Design review of the part shown in the three views and the two pictorial views. Dimensions are in mm from the part's minimum x, y and z. Coordinates: 2 decimals unless noted, no trailing zeros. Write each loop counter-clockwise with the first axis right and the second up, starting at its lowest first coordinate (ties: lowest second). Pieces come first, ordered by that corner, then holes. Notation, with made-up numbers: (-24.5, 27) -> (30.5, 27) arc R15 ccw to (30.5, 38) -> close; hole circle Ø1 at (48, -25.5). An arc over 180 degrees is marked (long way). Write item = value, one per line. Start each with the question number.
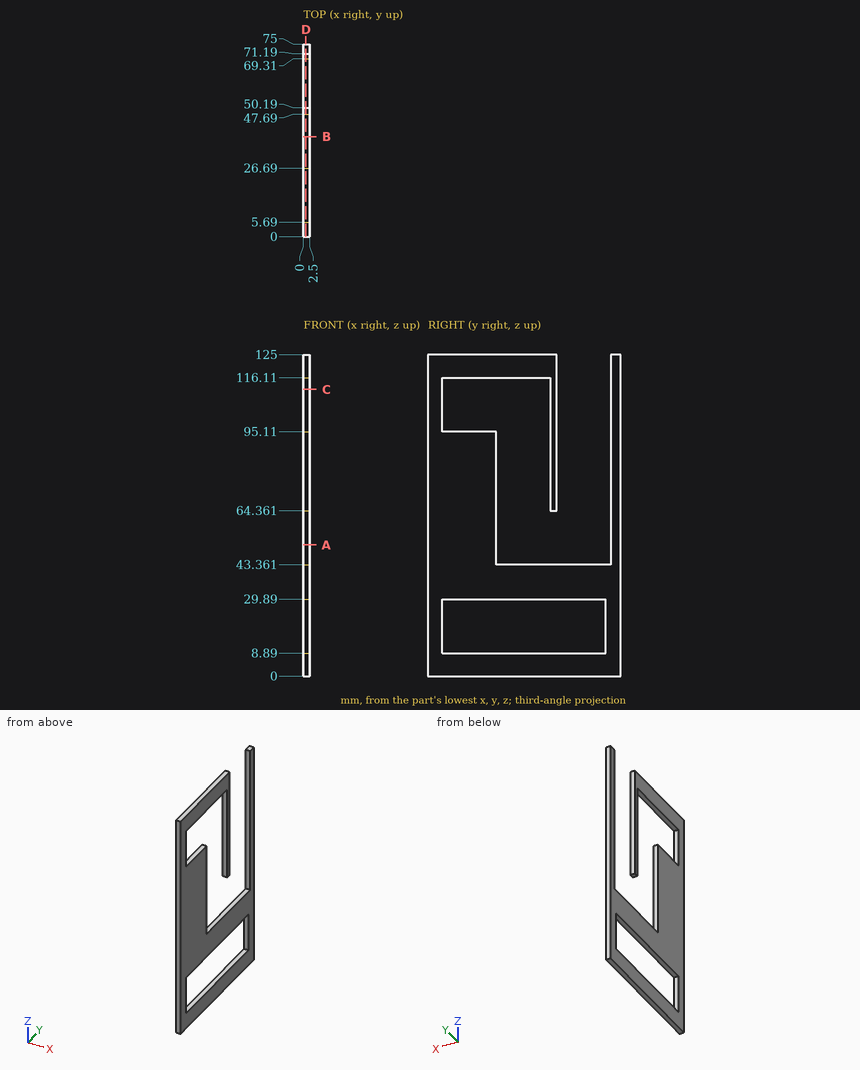
(1) Take a section at C-C, the plane z = 111.5. State the section outline as (x, y) points, then the cut area to 3 significant figures.
(2) Take a section at B-B, the plane y = 39. State the section outline as (x, z) points, then the cut area to 3 significant figures.
(3) Take a section at A-A, the plane z = 51. State the section outline as (x, y) points.
(4) For line 1 (Y direction, x = 2.45, z = 88.5); line 2 (Z direction, x = 1.3, y = 8); line 3 (Z direction, x = 0.8, y = 34.5), list the stretches that pass through material, from the lowest coordinate up.
(5) Take a section at D-D, the plane x = 1. State the section outline as (y, z) points, then the cut area to 3 significant figures.
(6) For pin 1 Ø8 at (y, z) = (40, 96.5) entering from -X, flat-tipped, find the tip position at first contact; note if it passes through.
Report:
q1.outline = (0, 0) -> (2.5, 0) -> (2.5, 5.69) -> (0, 5.69) -> close; (0, 47.69) -> (2.5, 47.69) -> (2.5, 50.19) -> (0, 50.19) -> close; (0, 71.19) -> (2.5, 71.19) -> (2.5, 75) -> (0, 75) -> close
q1.area = 30.0 mm2
q2.outline = (0, 0) -> (2.5, 0) -> (2.5, 8.89) -> (0, 8.89) -> close; (0, 29.89) -> (2.5, 29.89) -> (2.5, 43.36) -> (0, 43.36) -> close; (0, 116.11) -> (2.5, 116.11) -> (2.5, 125) -> (0, 125) -> close
q2.area = 78.1 mm2
q3.outline = (0, 0) -> (2.5, 0) -> (2.5, 26.69) -> (0, 26.69) -> close; (0, 71.19) -> (2.5, 71.19) -> (2.5, 75) -> (0, 75) -> close
q4.line_1 = 0 to 26.69, 47.69 to 50.19, 71.19 to 75
q4.line_2 = 0 to 8.89, 29.89 to 95.11, 116.11 to 125
q4.line_3 = 0 to 8.89, 29.89 to 43.36, 116.11 to 125
q5.outline = (0, 0) -> (75, 0) -> (75, 125) -> (71.19, 125) -> (71.19, 43.36) -> (26.69, 43.36) -> (26.69, 95.11) -> (5.69, 95.11) -> (5.69, 116.11) -> (47.69, 116.11) -> (47.69, 64.36) -> (50.19, 64.36) -> (50.19, 125) -> (0, 125) -> close; hole (5.69, 8.89) -> (69.31, 8.89) -> (69.31, 29.89) -> (5.69, 29.89) -> close
q5.area = 4,300 mm2
q6.pin_1 = through
